The model under review builds one solid part; all positions refer to its coordinate system, in mm. A direction names the side the tool comes from. Give positions to 0.01 mm unless a question says otherwise; leave off trailing zeros. Order: outer loops, then holes, each group sorted by start corner. A loop starts at its lowest first (then second) coordinate and runs counter-clockwise, first axis right, second up. Notation, with made-up numbers: (58.25, 59.25) - (75.25, 59.25) arc R21 cw to (75.25, 79.25) - close; hole circle Ø10 at (25, 61). An arc over 180 degrees is marked (long way). Use CSV: the item, a comma, the result in double quotes. Start each with the question number.
1. Draft analysis for pull direction Z (two halves, no side actions). For faces 5 (the cylindrical face through (-12.395, 63.908, 3.903)), 6 (the flat face through (-5, 52, -6)), 7 (the cylindrical face through (-41.42, -10.49, 10.72)), 8 (the flat face through (0, 54, -15)), state which applies: released by +Z, released by -Z, zero draft, split by the parting line, or undercut.
2. Machinability: for faces 1 (the cylindrical face through (-12.932, 62.659, -5.362)), 2 (the conical face through (35.142, -10.467, 10.239)), 3 (the flat face through (-48, 23, 0)), 4 (the flat face through (35, 17, 0)), which of the approach directions +Z, -Z, +X, -X, +Y, -Y give a long, thin tool a straight path to every point of the face, cutting with its end or side? Answer none if there is none.
3. To check wall thickness, follow line 1 (Z direction, x = -42, y = 0) (3 decimals); line 2 (X direction, y = 9, z = -4); line 3 (Z direction, x = -35.9, y = 0). State the ranges of each line that lie inside material, in increasing order. Write a range as [from, to].
4. Take a section at A-A, the plane y = 25. State the section outline as (x, z) points.
5. Take a section at D-D, the plane y = -4. Count the separate pieces of the cut face and the enclosed holes in it, then the cut area to 3 significant figures.
6. Take a section at C-C, the plane x = -17. State the section outline as (y, z) points, then the cut area to 4 significant figures.
7. For pin 1 (13 mm diameter, centred on x = -1.5, z = -4, fed in from +Y); pin 2 (12 mm diameter, centred on y = 47, z = -6.5, fed in from -X); pin 3 (3 mm diameter, centred on y = 52.5, z = 7, fed in from +X), all flat-tipped, find the tip position at first contact; note any pin that passes through.
8. Take a section at B-B, the plane x = 0. State the section outline as (y, z) points (3 decimals).
```python
from build123d import *

# Parameters (mm, degrees)
F0_W          = 30
F0_H          = 13
F0_W_2        = 13
F0_H_2        = 30
F1_DEPTH      = 15
F1_DEPTH_BACK = 15
F2_R          = 14.99999
F3_R          = 28
F4_R          = 12.995
F4_R_2        = 7.5
F5_DEPTH      = 11
F6_DEPTH      = 13
F7_R          = 12.995
F7_R_2        = 7.5
F8_DEPTH      = 11
F9_DEPTH      = 13
F10_START     = -1.7
F7_R_3        = 14
F10_DEPTH     = 1.3
F12_SIZE      = 0.5


# Not quite as in the source:
# - a fillet or chamfer is up to 0.001 mm smaller than in the source, because OpenCascade refuses the exact size


with BuildPart() as f1:
    # F0 (on Top) → F1 (new body, two sides)
    with BuildSketch(Plane.XY) as f1_sk:
        with Locations((0, 58.5)):
            Rectangle(F0_W, F0_H)
        Polygon((-48, 15), (-35, 15), (-35, 52), (-15, 52), (-15, 65), (-48, 65), align=None)
        with Locations((-41.5, 0)):
            Rectangle(F0_W_2, F0_H_2)
        Polygon((35, 52), (35, 15), (48, 15), (48, 65), (15, 65), (15, 52), align=None)
        with Locations((41.5, 0)):
            Rectangle(F0_W_2, F0_H_2)
    extrude(amount=F1_DEPTH)
    extrude(f1_sk.sketch, amount=-F1_DEPTH_BACK)

    # F2 (radius 15 in the source; OpenCascade refuses exactly that, so slightly less here)
    f2_edges = [f1.edges().sort_by_distance(p)[0] for p in [
        (-41.5, -15, 15),
        (-41.5, -15, -15),
        (41.5, -15, 15),
        (41.5, -15, -15),
        (-35, 52, 0),
        (35, 52, 0),
    ]]
    fillet(f2_edges, radius=F2_R)

    # F3
    f3_edges = [f1.edges().sort_by_distance(p)[0] for p in [
        (48, 65, 0),
        (-48, 65, 0),
    ]]
    fillet(f3_edges, radius=F3_R)

    # F4 (on face) → F5 (cut)
    with BuildSketch(Plane(origin=(-48, 0, 0), x_dir=(0, -1, 0), z_dir=(-1, 0, 0))):
        Circle(F4_R)
        Circle(F4_R_2, mode=Mode.SUBTRACT)
        Circle(F4_R_2)
    extrude(amount=-F5_DEPTH, mode=Mode.SUBTRACT)

    # F4 (on face) → F6 (cut)
    with BuildSketch(Plane(origin=(-48, 0, 0), x_dir=(0, -1, 0), z_dir=(-1, 0, 0))):
        Circle(F4_R_2)
    extrude(amount=-F6_DEPTH, mode=Mode.SUBTRACT)

    # F7 (on face) → F8 (cut)
    with BuildSketch(Plane(origin=(0, 65, 0), x_dir=(-1, 0, 0), z_dir=(0, 1, 0))):
        Circle(F7_R)
        Circle(F7_R_2, mode=Mode.SUBTRACT)
        Circle(F7_R_2)
    extrude(amount=-F8_DEPTH, mode=Mode.SUBTRACT)

    # F7 (on face) → F9 (cut)
    with BuildSketch(Plane(origin=(0, 65, 0), x_dir=(-1, 0, 0), z_dir=(0, 1, 0))):
        Circle(F7_R_2)
    extrude(amount=-F9_DEPTH, mode=Mode.SUBTRACT)

    # F7 (on face) → F10 (cut)
    with BuildSketch(Plane(origin=(0, 65, 0), x_dir=(-1, 0, 0), z_dir=(0, 1, 0)).offset(F10_START)):
        Circle(F7_R_3)
        Circle(F7_R, mode=Mode.SUBTRACT)
    extrude(amount=-F10_DEPTH, mode=Mode.SUBTRACT)

    # F11: F1 across plane


with BuildPart() as f1_1:
    add(f1.part)
    add(f1.part.mirror(Plane.YZ), mode=Mode.INTERSECT)

    # F12
    f12_edges = [f1_1.edges().sort_by_distance(p)[0] for p in [
        (-30.606605, 47.606605, 15),
        (0, 65, -15),
        (-48, 12.995, 0),
        (-37, 7.5, 0),
        (48, 12.995, 0),
        (37, 7.5, 0),
        (12.995, 65, 0),
        (7.5, 54, 0),
        (-48, 18.499995, 15),
        (-48, -10.606605, 10.606605),
        (-48, 18.499995, -15),
        (-48, -15, 0),
        (-48, -10.606605, -10.606605),
        (-35, 18.5, 15),
        (-35, -10.606605, 10.606605),
        (-35, -15, 0),
        (-35, 18.5, -15),
        (-35, -10.606605, -10.606605),
        (-30.606605, 47.606605, -15),
        (0, 52, 15),
        (0, 52, -15),
        (0, 65, 15),
        (39.79899, 56.79899, 15),
        (39.79899, 56.79899, -15),
        (48, 18.499995, 15),
        (48, -10.606605, 10.606605),
        (48, -15, 0),
        (48, 18.499995, -15),
        (48, -10.606605, -10.606605),
        (35, 18.5, 15),
        (35, -10.606605, 10.606605),
        (35, 18.5, -15),
        (35, -15, 0),
        (35, -10.606605, -10.606605),
        (30.606605, 47.606605, -15),
        (30.606605, 47.606605, 15),
        (-39.79899, 56.79899, -15),
        (-39.79899, 56.79899, 15),
    ]]
    chamfer(f12_edges, length=F12_SIZE)


solid = f1_1.part
```
Determined:
1,face 5,"undercut"
1,face 6,"zero draft"
1,face 7,"released by +Z"
1,face 8,"released by -Z"
2,face 1,"none"
2,face 2,"+Z, -Y"
2,face 3,"+Z, -Z, -X, +Y, -Y"
2,face 4,"+Z, -Z, -Y"
3,line 1,"z = [-15, -12.995], [12.995, 15]"
3,line 2,"x = [-37, -35], [35, 37]"
3,line 3,"z = [-15, -7.5], [7.5, 15]"
4,outline,"(-48, -14.5) - (-47.5, -15) - (-35.5, -15) - (-35, -14.5) - (-35, 14.5) - (-35.5, 15) - (-47.5, 15) - (-48, 14.5) - close; (35, -14.5) - (35.5, -15) - (47.5, -15) - (48, -14.5) - (48, 14.5) - (47.5, 15) - (35.5, 15) - (35, 14.5) - close"
5,separate pieces,"4"
5,enclosed holes,"0"
5,area,"155 mm²"
6,outline,"(52, -14.5) - (52.5, -15) - (64.5, -15) - (65, -14.5) - (65, 14.5) - (64.5, 15) - (52.5, 15) - (52, 14.5) - close"
6,area,"389.5 mm²"
7,pin 1,"stops at y = 54"
7,pin 2,"stops at x = -47.71"
7,pin 3,"stops at x = 44.25"
8,outline,"(52, -14.5) - (52.5, -15) - (64.5, -15) - (65, -14.5) - (65, -13.495) - (64.5, -12.995) - (63.3, -12.995) - (63.3, -14) - (62, -14) - (62, -12.995) - (54, -12.995) - (54, -8) - (53.5, -7.5) - (52, -7.5) - close; (52, 7.5) - (53.5, 7.5) - (54, 8) - (54, 12.995) - (62, 12.995) - (62, 14) - (63.3, 14) - (63.3, 12.995) - (64.5, 12.995) - (65, 13.495) - (65, 14.5) - (64.5, 15) - (52.5, 15) - (52, 14.5) - close"
